Drawing for the job (mm, zero at the part's lowest x, y, z). Round coordinates to 2 decimals unless told otherwise and drop trailing zeros. Write each loop counter-clockwise with the first axis right and the second up, starting at its lowest first coordinate (ties: lowest second). Pieces come first, ordered by that corner, then holes. Notation, with made-up numbers: (-33, -6.5) - (5, -6.5) arc R17 ccw to (5, 4.5) - close; hole circle Ø6 at (-10, 75.25). An arc over 180 degrees is marked (long way). One line per question, with ' | ' between items.
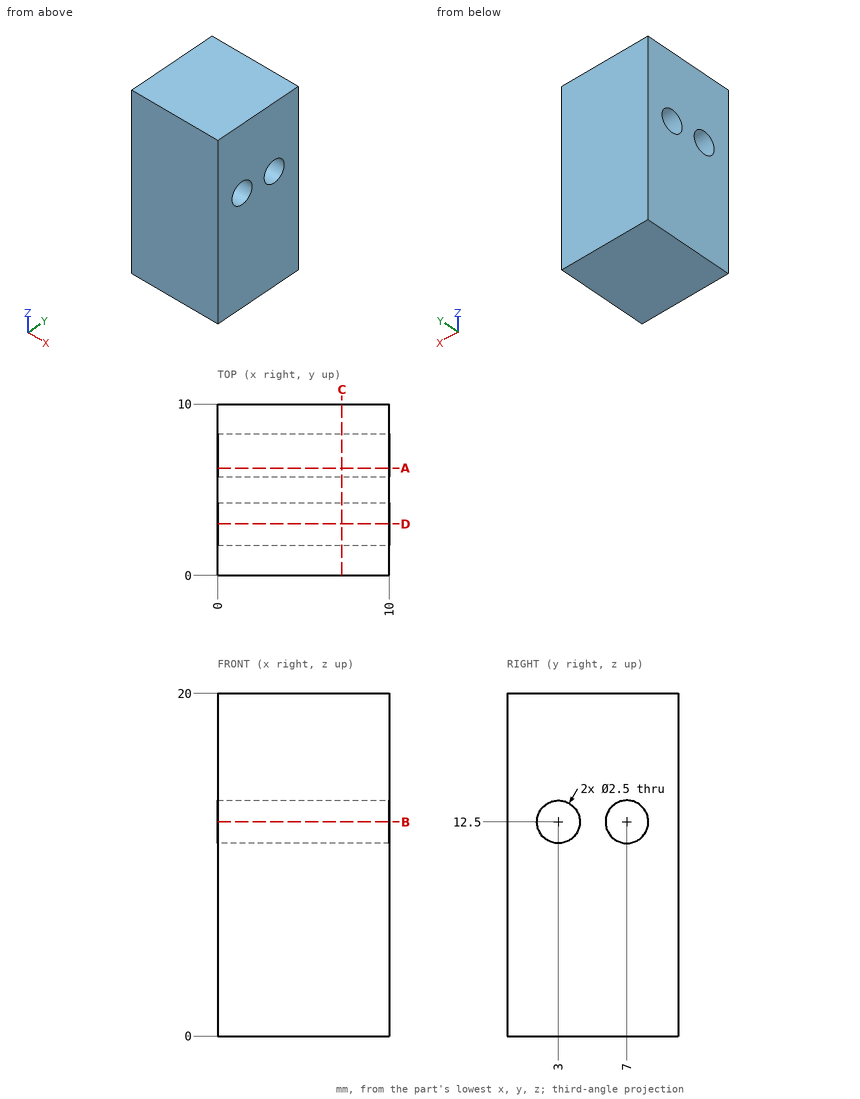
Q1. Saw through at C-C, the plane x = 7.25. List the corners of the cut face in (y, z), then the cut area to 3 significant figures.
Found:
outline: (0, 0) - (10, 0) - (10, 20) - (0, 20) - close; hole circle Ø2.5 at (3, 12.5); hole circle Ø2.5 at (7, 12.5) | area: 190 mm^2
Q2. Saw through at D-D, the plane y = 3. List the corners of the cut face in (x, z), then the cut area to 3 significant figures.
Found:
outline: (0, 0) - (10, 0) - (10, 11.25) - (0, 11.25) - close; (0, 13.75) - (10, 13.75) - (10, 20) - (0, 20) - close | area: 175 mm^2
Q3. Drill centre lines: L1, parallel to Y at x = 7.25, z = 12.5; L2, parallel to Z at x = 6.5, y = 3; L3, parallel to Y at x = 4.25, z = 13.25. Where is each one in solid material? Low to high. Write a range as from..to.
Found:
L1: 0..1.75, 4.25..5.75, 8.25..10 | L2: 0..11.25, 13.75..20 | L3: 0..2, 4..6, 8..10
Q4. Saw through at B-B, the plane z = 12.5. List the corners of the cut face in (x, y), then the cut area to 3 significant figures.
Found:
outline: (0, 0) - (10, 0) - (10, 1.75) - (0, 1.75) - close; (0, 4.25) - (10, 4.25) - (10, 5.75) - (0, 5.75) - close; (0, 8.25) - (10, 8.25) - (10, 10) - (0, 10) - close | area: 50.0 mm^2
Q5. Drop flat-ended pins along their axis: pin 1 (2 mm diameter, centred on y = 7, z = 12.5, fed in from +X); pin 2 (5 mm diameter, centred on y = 3.5, z = 12, fed in from +X). Give the stop position or say it passes through.
Found:
pin 1: through | pin 2: x = 10
Q6. Saw through at A-A, the plane y = 6.25. List the corners of the cut face in (x, z).
Found:
outline: (0, 0) - (10, 0) - (10, 11.5) - (0, 11.5) - close; (0, 13.5) - (10, 13.5) - (10, 20) - (0, 20) - close
